The model under review builds one solid part; all positions refer to its coordinate system, in mm. Face numbers are marked on the shaded views. A direction names the side the tool comes from. Coordinates: 2 decimals unless noted, no trailing zeros. Loops run counter-clockwise (first coordinate to the right, second up) from the corner with the lowest first, then second, coordinate; pieces in that order, holes last. Notation, with made-up numbers: M 41.25,-27.75 L 64.25,-27.75 A34 cw 64.25,3.25 Z; hole C 36,56 d3. An arc over 180 degrees is marked long. Use CSV: the item, a comma, the result in double quotes. Start each with the question number.
1. Add section D-D, the plane z = 1.5. Write out the cut boundary in (x, y).
2. Draft analysis for pull direction Y (two halves, no side actions). For the marked faces 1, 2 and 3, state which applies: +Y half, -Y half, draft (parallel to the pull), parting line (faces both ways), or undercut.
3. For L1, parallel to Y at x = 0, z = 1.4; L2, parallel to Z at x = 6, y = 9.5; L3, parallel to Y at x = 12.5, z = -2.55, list the stretches that pass through material, from the lowest coordinate up.
4. Clearance check with flat-ended pins moving along their axes: P1, Ø3, axis at x = 1.5, y = -12.5, coming from the +Z side (3 decimals); P2, Ø2, axis at y = 2.5, z = -2, coming from the -X side; P3, Ø4, axis at x = 10.5, z = -1.5, coming from the +Y side. State where each tip first meets the part, or that it passes through.
5. Tool access review of the marked faces 4, 5 and 6: name each direction out of +Z, -Z, +X, -X, +Y, -Y from which nothing blocks a thin tool from reaching the whole face with its end or side.
6. Add section B-B, the plane x = 6. Write out the cut boundary in (y, z), then the cut area to 3 significant figures.
7. Add section A-A, the plane z = -0.5. Write out the cut boundary in (x, y) (3 decimals).
from build123d import *

# Parameters (mm, degrees)
SKETCH1_R             = 8.7
BOSS_EXTRUDE1_DEPTH   = 2.54
SKETCH2_R             = 2
BOSS_EXTRUDE2_DEPTH   = 3
SKETCH3_R             = 16.25
BOSS_EXTRUDE3_DEPTH   = 3.81
CUT_EXTRUDE1_DEPTH    = 1.905
F_4_CLEARANCE_HOLE1_D = 2.9464
CIRPATTERN1_COUNT     = 4
SKETCH8_R             = 1.75
CUT_EXTRUDE2_DEPTH    = 2.5
SKETCH9_R             = 3.5
CUT_EXTRUDE3_DEPTH    = 24.629959797


with BuildPart() as part:
    # Sketch1 → Boss-Extrude1 (new body)
    with BuildSketch(Plane.XY):
        Circle(SKETCH1_R)
    extrude(amount=BOSS_EXTRUDE1_DEPTH)

    # Sketch2 → Boss-Extrude2 (add)
    with BuildSketch(Plane.XY.offset(2.54)):
        with Locations((0, 6)):
            Circle(SKETCH2_R)
        with Locations((6, 0)):
            Circle(SKETCH2_R)
        with Locations((0, -6)):
            Circle(SKETCH2_R)
        with Locations((-6, 0)):
            Circle(SKETCH2_R)
    extrude(amount=BOSS_EXTRUDE2_DEPTH)

    # Sketch3 → Boss-Extrude3 (add)
    with BuildSketch(Plane(origin=(0, 0, 0), x_dir=(-1, 0, 0), z_dir=(0, 0, -1))):
        with Locations(Location((0, 0, 0), (0, 0, 180))):
            Circle(SKETCH3_R)
    extrude(amount=BOSS_EXTRUDE3_DEPTH)

    # Sketch4 → Cut-Extrude1 (cut)
    with BuildSketch(Plane.XY):
        Polygon((-12.5, 3.666174209), (-15.675, 1.833087105), (-15.675, -1.833087105), (-12.5, -3.666174209), (-9.325, -1.833087105), (-9.325, 1.833087105), align=None)
    cut_extrude1 = extrude(amount=-CUT_EXTRUDE1_DEPTH, mode=Mode.SUBTRACT)

    # #4 Clearance Hole1 (through all)
    with Locations(Plane.XY.offset(-1.905)):
        with Locations((-12.5, 0)):
            f_4_clearance_hole1 = Hole(F_4_CLEARANCE_HOLE1_D / 2)

    # CirPattern1: Cut-Extrude1, #4 Clearance Hole1 ×4 about axis
    cirpattern1_axis = Axis((0, 0, 0), (0, 0, 1))
    add([cut_extrude1.rotate(cirpattern1_axis, i * 360 / CIRPATTERN1_COUNT) for i in range(1, CIRPATTERN1_COUNT)], mode=Mode.SUBTRACT)
    add([f_4_clearance_hole1.rotate(cirpattern1_axis, i * 360 / CIRPATTERN1_COUNT) for i in range(1, CIRPATTERN1_COUNT)], mode=Mode.SUBTRACT)

    # Sketch8 → Cut-Extrude2 (cut)
    with BuildSketch(Plane.XY.offset(2.54)):
        Circle(SKETCH8_R)
    extrude(amount=-CUT_EXTRUDE2_DEPTH, mode=Mode.SUBTRACT)

    # Sketch9 → Cut-Extrude3 (cut, through all)
    with BuildSketch(Plane.XY.offset(0.04)):
        Circle(SKETCH9_R)
    extrude(amount=-CUT_EXTRUDE3_DEPTH, mode=Mode.SUBTRACT)


solid = part.part
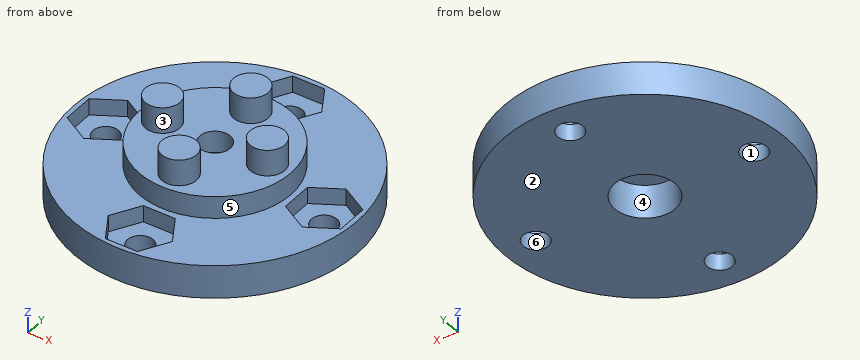
Computed:
1,outline,"C 0,0 d17.4; hole C 0,0 d3.5"
2,face 1,"undercut"
2,face 2,"draft"
2,face 3,"parting line"
3,L1,"y = -8.7 to -1.75, 1.75 to 8.7"
3,L2,"z = -3.81 to 0"
3,L3,"y = -10.38 to -1.47, 1.47 to 10.38"
4,P1,"stops at z = -1.905"
4,P2,"stops at x = -16.18"
4,P3,"stops at y = 13.85"
5,face 4,"-Z"
5,face 5,"+Z"
5,face 6,"+Z, -Z"
6,outline,"M -15.1,-3.81 L 15.1,-3.81 L 15.1,0 L 6.3,0 L 6.3,2.54 L 2,2.54 L 2,5.54 L -2,5.54 L -2,2.54 L -6.3,2.54 L -6.3,0 L -15.1,0 Z"
6,area,"159 mm^2"
7,outline,"C 0,0 d32.5; hole M -15.675,-1.833 L -12.5,-3.666 L -9.325,-1.833 L -9.325,1.833 L -12.5,3.666 L -15.675,1.833 Z; hole M -3.666,-12.5 L -1.833,-15.675 L 1.833,-15.675 L 3.666,-12.5 L 1.833,-9.325 L -1.833,-9.325 Z; hole M -3.666,12.5 L -1.833,9.325 L 1.833,9.325 L 3.666,12.5 L 1.833,15.675 L -1.833,15.675 Z; hole C 0,0 d7; hole M 9.325,-1.833 L 12.5,-3.666 L 15.675,-1.833 L 15.675,1.833 L 12.5,3.666 L 9.325,1.833 Z"
